Design review of the part built by this model. Coordinates are the model's own, in mm. A direction names the side the tool comes from. Coordinates: 2 decimals unless noted, no trailing zeros. Loops run counter-clockwise (first coordinate to the right, second up) from the corner with the lowest first, then second, coordinate; pieces in that order, holes last. Notation, with made-up numbers: (61, -35.5) -> (103, -35.5) arc R17 cw to (103, -25.5) -> close; hole circle Ø6 at (18, 67.5). An arc over 180 degrees is marked (long way). Answer as a JSON object with one key per item and string values.
```python
from build123d import *

# Parameters (mm, degrees)
F2_SIZE = 0.3


with BuildPart() as f1:
    # F0 (on Front) → F1 (revolve)
    with BuildSketch(Plane.XZ):
        Polygon((4.2, 3), (3, 3), (3, -3), (4.079062, -3), (4.079062, -2.7), (8.3, -2.7), (8.3, -3), (9.5, -3), (9.5, 3), (8.3, 3), (8.3, 2.7), (4.2, 2.7), align=None)
    revolve(axis=Axis((0, 0, 0), (0, 0, -1)))

    # F2
    f2_edges = [f1.edges().sort_by_distance(p)[0] for p in [
        (-9.5, 0, 3),
        (-9.5, 0, -3),
        (-3, 0, 3),
        (-3, 0, -3),
    ]]
    chamfer(f2_edges, length=F2_SIZE)


solid = f1.part
```
1) For faces 4 (the flat face through (4, 2, -2.7)), 5 (the flat face through (-5, -7, 3)), list the 3-axis set-ups (+Z, -Z, +X, -X, +Y, -Y) from which the entire face can be reached by the end or side of a thin tool; tool diameter is ignored.
Completed:
{"face 4": "-Z", "face 5": "+Z, +X, -X, +Y, -Y"}
2) Wall thickness on probe 1 along Y at (x, z) = (0, -0.2); probe 2 along X at (y, z) = (0, -2.75); probe 3 along Y at (x, z) = (0, -2.9): over which ranges is each line inside the solid? List them lowest first.
Completed:
{"probe 1": "-9.5 to -3, 3 to 9.5", "probe 2": "-9.45 to -8.3, -4.08 to -3.05, 3.05 to 4.08, 8.3 to 9.45", "probe 3": "-9.3 to -8.3, -4.08 to -3.2, 3.2 to 4.08, 8.3 to 9.3"}
3) The part is to be moulded in two halves that separate along X. For faces 1 (the flat face through (-4, -2, 2.7)), 2 (the flat face through (2, 3, -3)), 3 (the cylindrical face through (4.38, 8.43, 0.04)), say which applies: pulls with the +X half, pulls with the -X half, needs draft (parallel to the pull), parting line crosses it, or undercut.
Completed:
{"face 1": "undercut", "face 2": "needs draft", "face 3": "parting line crosses it"}
4) Clearance check with flat-ended pins moving along their axes: pin 1 Ø8 at (x, y) = (0, 0) entering from -Z; pin 2 Ø3 at (x, z) = (-5, 2.5) entering from +Y; pin 3 Ø1.5 at (y, z) = (-6, 2.5) entering from -X; pin 4 Ø1.5 at (x, y) = (2.5, 6) entering from -Z. State where each tip first meets the part, or that it passes through.
Completed:
{"pin 1": "z = -3", "pin 2": "y = 8.83", "pin 3": "x = -7.92", "pin 4": "z = -2.7"}
5) Add section C-C, the plane z = -2.35. Give the boundary of the cut face in (x, y).
Completed:
{"outline": "circle Ø19 at (0, 0); hole circle Ø6 at (0, 0)"}
